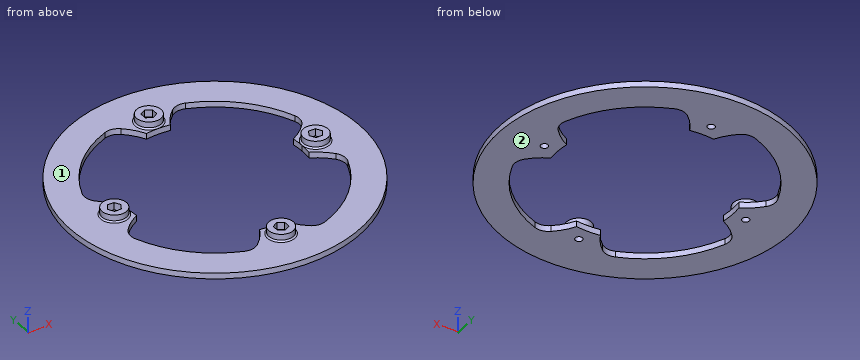
```python
from build123d import *

# Parameters (mm, degrees)
F0_R     = 100
F0_R_2   = 2.5
F1_DEPTH = 4
F2_R     = 8.5
F3_DEPTH = 5
F4_R     = 10
F5_R     = 0.99999


# Not quite as in the source:
# - a fillet or chamfer is up to 0.001 mm smaller than in the source, because OpenCascade refuses the exact size


with BuildPart() as f1:
    # F0 (on Top) → F1 (new body)
    with BuildSketch(Plane.XY):
        Circle(F0_R)
        with BuildLine():
            ThreePointArc((22.8257041117, 75.7052949069), (55.9120042797, 55.9120042797), (75.7052949069, 22.8257041117))
            ThreePointArc((75.7052949069, 22.8257041117), (78.2254331665, 11.536292778), (79.0715147518, 0))
            ThreePointArc((79.0715147518, 0), (78.2254331665, -11.536292778), (75.7052949069, -22.8257041117))
            ThreePointArc((75.7052949069, -22.8257041117), (55.9120042797, -55.9120042797), (22.8257041117, -75.7052949069))
            ThreePointArc((22.8257041117, -75.7052949069), (0, -79.0715147518), (-22.8257041117, -75.7052949069))
            ThreePointArc((-22.8257041117, -75.7052949069), (-55.9120042797, -55.9120042797), (-75.7052949069, -22.8257041117))
            ThreePointArc((-75.7052949069, -22.8257041117), (-79.0715147518, 0), (-75.7052949069, 22.8257041117))
            ThreePointArc((-75.7052949069, 22.8257041117), (-55.9120042797, 55.9120042797), (-22.8257041117, 75.7052949069))
            ThreePointArc((-22.8257041117, 75.7052949069), (0, 79.0715147518), (22.8257041117, 75.7052949069))
        make_face(mode=Mode.SUBTRACT)
        with BuildLine():
            ThreePointArc((-8.3091100857, 59.9266942988), (0, 60.5), (8.3091100857, 59.9266942988))
            ThreePointArc((8.3091100857, 59.9266942988), (14.4468681442, 68.8469104297), (22.8257041117, 75.7052949069))
            ThreePointArc((22.8257041117, 75.7052949069), (0, 79.0715147518), (-22.8257041117, 75.7052949069))
            ThreePointArc((-22.8257041117, 75.7052949069), (-14.4468681442, 68.8469104297), (-8.3091100857, 59.9266942988))
        make_face()
        Polygon((0.2799602618, 74.6188021535), (4.2799602618, 72.3094010768), (4.2799602618, 67.6905989232), (0.2799602618, 65.3811978465), (-3.7200397382, 67.6905989232), (-3.7200397382, 72.3094010768), align=None, mode=Mode.SUBTRACT)
        with BuildLine():
            ThreePointArc((-59.9266942988, -8.3091100857), (-60.5, 0), (-59.9266942988, 8.3091100857))
            ThreePointArc((-59.9266942988, 8.3091100857), (-68.8469104297, 14.4468681442), (-75.7052949069, 22.8257041117))
            ThreePointArc((-75.7052949069, 22.8257041117), (-79.0715147518, 0), (-75.7052949069, -22.8257041117))
            ThreePointArc((-75.7052949069, -22.8257041117), (-68.8469104297, -14.4468681442), (-59.9266942988, -8.3091100857))
        make_face()
        Polygon((-65.3811978465, 0.2799602618), (-67.6905989232, -3.7200397382), (-72.3094010768, -3.7200397382), (-74.6188021535, 0.2799602618), (-72.3094010768, 4.2799602618), (-67.6905989232, 4.2799602618), align=None, mode=Mode.SUBTRACT)
        with BuildLine():
            ThreePointArc((59.9266942988, 8.3091100857), (60.3565033989, 4.1644324296), (60.5, 0))
            ThreePointArc((60.5, 0), (60.3565033989, -4.1644324296), (59.9266942988, -8.3091100857))
            ThreePointArc((59.9266942988, -8.3091100857), (68.8469104297, -14.4468681442), (75.7052949069, -22.8257041117))
            ThreePointArc((75.7052949069, -22.8257041117), (78.2254331665, -11.536292778), (79.0715147518, 0))
            ThreePointArc((79.0715147518, 0), (78.2254331665, 11.536292778), (75.7052949069, 22.8257041117))
            ThreePointArc((75.7052949069, 22.8257041117), (68.8469104297, 14.4468681442), (59.9266942988, 8.3091100857))
        make_face()
        Polygon((74.6188021535, -0.2799602618), (72.3094010768, -4.2799602618), (67.6905989232, -4.2799602618), (65.3811978465, -0.2799602618), (67.6905989232, 3.7200397382), (72.3094010768, 3.7200397382), align=None, mode=Mode.SUBTRACT)
        with BuildLine():
            ThreePointArc((22.8257041117, -75.7052949069), (14.4468681442, -68.8469104297), (8.3091100857, -59.9266942988))
            ThreePointArc((8.3091100857, -59.9266942988), (0, -60.5), (-8.3091100857, -59.9266942988))
            ThreePointArc((-8.3091100857, -59.9266942988), (-14.4468681442, -68.8469104297), (-22.8257041117, -75.7052949069))
            ThreePointArc((-22.8257041117, -75.7052949069), (0, -79.0715147518), (22.8257041117, -75.7052949069))
        make_face()
        Polygon((-0.2799602618, -74.6188021535), (-4.2799602618, -72.3094010768), (-4.2799602618, -67.6905989232), (-0.2799602618, -65.3811978465), (3.7200397382, -67.6905989232), (3.7200397382, -72.3094010768), align=None, mode=Mode.SUBTRACT)
        Polygon((-72.3094010768, -3.7200397382), (-67.6905989232, -3.7200397382), (-65.3811978465, 0.2799602618), (-67.6905989232, 4.2799602618), (-72.3094010768, 4.2799602618), (-74.6188021535, 0.2799602618), align=None)
        with Locations((-70, 0)):
            Circle(F0_R_2, mode=Mode.SUBTRACT)
        Polygon((-4.2799602618, -67.6905989232), (-4.2799602618, -72.3094010768), (-0.2799602618, -74.6188021535), (3.7200397382, -72.3094010768), (3.7200397382, -67.6905989232), (-0.2799602618, -65.3811978465), align=None)
        with Locations((0, -70)):
            Circle(F0_R_2, mode=Mode.SUBTRACT)
        Polygon((67.6905989232, -4.2799602618), (72.3094010768, -4.2799602618), (74.6188021535, -0.2799602618), (72.3094010768, 3.7200397382), (67.6905989232, 3.7200397382), (65.3811978465, -0.2799602618), align=None)
        with Locations((70, 0)):
            Circle(F0_R_2, mode=Mode.SUBTRACT)
        Polygon((4.2799602618, 67.6905989232), (4.2799602618, 72.3094010768), (0.2799602618, 74.6188021535), (-3.7200397382, 72.3094010768), (-3.7200397382, 67.6905989232), (0.2799602618, 65.3811978465), align=None)
        with Locations((0, 70)):
            Circle(F0_R_2, mode=Mode.SUBTRACT)
    extrude(amount=F1_DEPTH)

    # F2 (on face) → F3 (join)
    with BuildSketch(Plane.XY.offset(4)):
        with Locations((-70, 0)):
            Circle(F2_R)
        Polygon((-67.7365000122, -4.0261521504), (-72.3550000478, -3.9733245662), (-74.6185000357, 0.0528275843), (-72.2634999878, 4.0261521504), (-67.6449999522, 3.9733245662), (-65.3814999643, -0.0528275843), align=None, mode=Mode.SUBTRACT)
        with Locations((0, 70)):
            Circle(F2_R)
        Polygon((-4.0261521504, 67.7365000122), (-3.9733245662, 72.3550000478), (0.0528275843, 74.6185000357), (4.0261521504, 72.2634999878), (3.9733245662, 67.6449999522), (-0.0528275843, 65.3814999643), align=None, mode=Mode.SUBTRACT)
        with Locations((70, 0)):
            Circle(F2_R)
        Polygon((67.7365000122, 4.0261521504), (72.3550000478, 3.9733245662), (74.6185000357, -0.0528275843), (72.2634999878, -4.0261521504), (67.6449999522, -3.9733245662), (65.3814999643, 0.0528275843), align=None, mode=Mode.SUBTRACT)
        with Locations((0, -70)):
            Circle(F2_R)
        Polygon((4.0261521504, -67.7365000122), (3.9733245662, -72.3550000478), (-0.0528275843, -74.6185000357), (-4.0261521504, -72.2634999878), (-3.9733245662, -67.6449999522), (0.0528275843, -65.3814999643), align=None, mode=Mode.SUBTRACT)
    extrude(amount=F3_DEPTH)

    # F4
    f4_edges = [f1.edges().sort_by_distance(p)[0] for p in [
        (-75.705295, 22.825704, 2),
        (-75.705295, -22.825704, 2),
        (75.705295, -22.825704, 2),
        (22.825704, -75.705295, 2),
        (-22.825704, -75.705295, 2),
        (75.705295, 22.825704, 2),
        (22.825704, 75.705295, 2),
        (-22.825704, 75.705295, 2),
    ]]
    fillet(f4_edges, radius=F4_R)

    # F5 (radius 1 in the source; OpenCascade refuses exactly that, so slightly less here)
    f5_edges = [f1.edges().sort_by_distance(p)[0] for p in [
        (-8.5, -70, 4),
        (-8.5, 70, 4),
        (-78.5, 0, 4),
        (61.5, 0, 4),
    ]]
    fillet(f5_edges, radius=F5_R)


solid = f1.part
```
Input: part model. Units: mm. Frame: model coordinates. Face numbers are marked on the shaded views. A direction names the side the tool comes from. Coordinates: 2 decimals unless noted, no trailing zeros. Order: outer loops, then holes, each group sorted by start corner. A loop starts at its lowest first (then second) coordinate and runs counter-clockwise, first axis right, second up. Notation, with made-up numbers: (-14, 42) - (1, 42) arc R22 ccw to (1, 50) - close; hole circle Ø6 at (12, 6). An arc over 180 degrees is marked (long way). Return JSON: item names as keys, results as strings.
Q1. Cut plane C-C (x = -86.5). Return loops of the section in (y, z).
The answers:
{"outline": "(-50.18, 0) - (50.18, 0) - (50.18, 4) - (-50.18, 4) - close"}
Q2. Access query for the marked faces 1 and 2. Directions: +Z, -Z, +X, -X, +Y, -Y. A direction counts if a zero-diameter tool reaches every point of the face in a straight line with its end or side. Return the directions, or none.
The answers:
{"face 1": "+Z", "face 2": "-Z, +X, -X, +Y, -Y"}
Q3. Ray query, probe 1 along Y at (x, z) = (0, 2.75); probe 2 along X at (y, z) = (-1, 2.75) (3 decimals). Return the intervals inside material, ascending.
The answers:
{"probe 1": "y = -100 to -72.5, -67.5 to -60.5, 60.5 to 67.5, 72.5 to 100", "probe 2": "x = -99.995 to -72.291, -67.709 to -60.492, 60.492 to 67.709, 72.291 to 99.995"}
Q4. First-contact query: pin 1 (1 mm diameter, centred on x = -74, y = 45, fed in from +Z). Flat tip, straight axial feed; report the tip coordinate or a pass-through.
The answers:
{"pin 1": "stops at z = 4"}
Q5. Cut plane A-A (z = 6.75). Return loops of the section in (x, y) (1 decimal), then the cut area to 3 significant figures.
The answers:
{"outline": "circle Ø17 at (-70, 0); circle Ø17 at (0, -70); circle Ø17 at (0, 70); circle Ø17 at (70, 0); hole (-74.6, 0.1) - (-72.4, -4) - (-67.7, -4) - (-65.4, -0.1) - (-67.6, 4) - (-72.3, 4) - close; hole (-4, -72.3) - (-0.1, -74.6) - (4, -72.4) - (4, -67.7) - (0.1, -65.4) - (-4, -67.6) - close; hole (-4, 67.7) - (-0.1, 65.4) - (4, 67.6) - (4, 72.3) - (0.1, 74.6) - (-4, 72.4) - close; hole (65.4, 0.1) - (67.6, -4) - (72.3, -4) - (74.6, -0.1) - (72.4, 4) - (67.7, 4) - close", "area": "686 mm2"}
Q6. Cut plane B-B (y = 83.5). Return loops of the section in (x, z) (3 decimals), then the cut area to 3 significant figures.
The answers:
{"outline": "(-55.025, 0) - (55.025, 0) - (55.025, 4) - (-55.025, 4) - close", "area": "440 mm2"}
